Autodesk Inventor part; units mm, degrees
ref_plane "YZ Plane" through (0, 0, 0) normal (1, 0, 0) x (0, 1, 0)
ref_plane "XZ Plane" through (0, 0, 0) normal (0, 1, 0) x (-1, 0, 0)
ref_plane "XY Plane" through (0, 0, 0) normal (0, 0, 1) x (1, 0, 0)
sketch "スケッチ1" plane through (0, 0, 0) normal (0, 1, 0) x (-1, 0, 0)
  circle A0 centre (0, 0) radius 122.5
  line L0 (0, 0) -> (21.2719, 120.6389)
  line L1 (21.2719, 120.6389) -> (-21.2719, -120.6389)
  line L2 (21.2719, 120.6389) -> (-41.166, -233.4643)
  arc A1 (21.2719, 120.6389) -> (0, 122.5) centre (0, 0) ccw
  arc A2 (-21.2719, -120.6389) -> (0, -122.5) centre (0, 0) ccw
  arc A3 (-41.8975, -115.1123) -> (-21.2719, -120.6389) centre (0, 0) ccw
  circle A4 centre (0, 0) radius 125
  circle A5 centre (0, 0) radius 145
  arc A6 (-42.7525, -117.4616) -> (-105.9051, -66.4011) centre (0, 0) ccw
  line L3 (0, 0) -> (-42.7525, -117.4616) construction
  line L4 (21.706, 123.101) -> (21.706, 123.101)
  line L5 (0, -145) -> (0, -265.735)
  line L6 (0, 0) -> (-41.8975, -115.1123)
  line L7 (-49.5929, -136.2554) -> (-41.8975, -115.1123)
  line L8 (-42.7525, -117.4616) -> (-231.4975, -48.764)
  line L9 (42.7525, 117.4616) -> (0, 0)
  line L10 (0, -145) -> (0, 145)
  line L11 (0, 0) -> (0, 250)
  circle A7 centre (0, 250) radius 20
  line L12 (113.4405, 52.5) -> (18.1505, 258.4)
  line L13 (0, 0) -> (185.4327, 0)
  line L14 (0, 0) -> (-259.4726, 94.4403)
  line L15 (42.7525, 117.4616) -> (-253.7236, 225.3701)
  line L16 (0, 125) -> (22.0409, 125)
  line L17 (21.2719, 120.6389) -> (25.179, 142.7971)
  line L18 (42.7525, 117.4616) -> (60.6365, 166.5974)
  line L19 (15, 170) -> (59.0618, 170)
  line L20 (15.9946, 175) -> (56.7478, 175)
  line L21 (0, 125) -> (-15, 125)
  line L22 (-15, 125) -> (-15, 275)
  line L23 (-15, 275) -> (0, 275)
  line L24 (0, 275) -> (0, 125)
  line L25 (0, 125) -> (15, 125)
  line L26 (15, 125) -> (15, 275)
  line L27 (15, 275) -> (0, 275)
  line L28 (0, 275) -> (0, 125)
  line L29 (15, 200) -> (15, 275)
  line L30 (15, 275) -> (-15, 275)
  line L31 (-15, 275) -> (-15, 150)
  line L32 (15, 170) -> (37.5, 170)
  line L33 (37.5, 170) -> (17.5, 170)
  line L34 (0, 0) -> (0, 250)
  line L35 (0, -125) -> (42.7525, 117.4616)
  line L36 (-42.7525, -117.4616) -> (0, 125)
  line L37 (0, -125) -> (-3.519, -144.9573)
  line L38 (42.7525, 117.4616) -> (49.5929, 136.2554)
  line L39 (0, 125) -> (3.519, 144.9573)
  line L40 (-42.7525, -117.4616) -> (-46.2715, -137.4189)
  line L41 (42.7525, 117.4616) -> (46.2715, 137.4189)
  line L42 (-3.519, -144.9573) -> (46.2715, 137.4189)
  line L43 (46.2715, 137.4189) -> (37.2054, 139.0175)
  line L44 (-12.5852, -143.3587) -> (-3.519, -144.9573)
  line L45 (-46.2715, -137.4189) -> (3.519, 144.9573)
  line L46 (3.519, 144.9573) -> (12.5852, 143.3587)
  line L47 (-37.2054, -139.0175) -> (-46.2715, -137.4189)
  line L48 (-27.6373, -142.3418) -> (-22.7132, -143.21)
  line L49 (-27.6373, -142.3418) -> (-22.7132, -143.21)
  line L50 (-22.7132, -143.21) -> (27.641, 142.363)
  line L51 (27.641, 142.363) -> (22.717, 143.2312)
  line L52 (22.717, 143.2312) -> (-27.6373, -142.3418)
  line L53 (12.5852, 143.3587) -> (-37.2054, -139.0175)
  line L54 (-12.5852, -143.3587) -> (37.2054, 139.0175)
  line L55 (-42.1294, -138.1492) -> (7.6611, 144.2269)
  line L56 (-7.6611, -144.2269) -> (42.1294, 138.1492)
  line L57 (12.5852, 143.3587) -> (7.6611, 144.2269)
  line L58 (7.6611, 144.2269) -> (23.8851, 236.2374)
  line L59 (23.8851, 236.2374) -> (28.8091, 235.3692)
  line L60 (28.8091, 235.3692) -> (12.5852, 143.3587)
  line L61 (22.717, 143.2312) -> (25.179, 142.7971)
  line L62 (25.179, 142.7971) -> (42.462, 240.8141)
  line L63 (42.462, 240.8141) -> (40, 241.2482)
  line L64 (40, 241.2482) -> (22.717, 143.2312)
  line L65 (42.1294, 138.1492) -> (37.2054, 139.0175)
  line L66 (37.2054, 139.0175) -> (45.9435, 188.5741)
  line L67 (45.9435, 188.5741) -> (50.8676, 187.7058)
  line L68 (50.8676, 187.7058) -> (42.1294, 138.1492)
  line L69 (25.179, 142.7971) -> (27.641, 142.363)
  line L70 (27.641, 142.363) -> (39.8383, 211.5375)
  line L71 (39.8383, 211.5375) -> (37.3763, 211.9716)
  line L72 (37.3763, 211.9716) -> (25.179, 142.7971)
  line L73 (15.9946, 175) -> (15, 175)
  line L74 (15, 175) -> (0, 175)
  line L75 (0, 175) -> (0, 170)
  line L76 (0, 170) -> (15, 170)
  line L77 (15, 170) -> (15, 175)
  line L78 (20, 175) -> (40, 175)
  line L79 (40, 175) -> (40, 245)
  line L80 (40, 245) -> (20, 245)
  line L81 (20, 245) -> (20, 175)
  line L82 (30, 175) -> (30, 118.7697)
  line L83 (0, 175) -> (45.1779, 175)
  line L84 (45.1779, 175) -> (45.1779, 200)
  line L85 (45.1779, 200) -> (0, 200)
  line L86 (0, 200) -> (0, 175)
  line L87 (0, 200) -> (50, 200)
  line L88 (50, 200) -> (50, 170)
  line L89 (50, 170) -> (0, 170)
  line L90 (0, 170) -> (0, 200)
  line L91 (50, 170) -> (0, 170)
  line L92 (0, 170) -> (0, 165)
  line L93 (0, 200) -> (-15, 200)
  line L94 (-15, 200) -> (-15, 180)
  line L95 (-15, 180) -> (0, 180)
  line L96 (0, 180) -> (0, 200)
  line L97 (0, 180) -> (-15, 180)
  line L98 (-15, 180) -> (-15, 175)
  line L99 (-15, 175) -> (0, 175)
  line L100 (0, 175) -> (0, 180)
  line L101 (0, 145) -> (-15, 145)
  line L102 (-15, 145) -> (-20.5, 145)
  line L103 (-20.5, 145) -> (-20.5, 200)
  line L104 (-20.5, 200) -> (-15, 200)
  line L105 (-15, 200) -> (-15, 145)
  line L106 (-20.5, 150) -> (-25, 150)
  line L107 (-25, 150) -> (-25, 180)
  line L108 (-25, 180) -> (-20.5, 180)
  line L109 (-20.5, 180) -> (-20.5, 150)
  line L110 (50, 175) -> (-15, 175)
  line L111 (-15, 175) -> (-15, 170)
  line L112 (50, 170) -> (50, 175)
  line L113 (-20.5, 165) -> (-25, 165)
  line L114 (-25, 165) -> (-25, 195)
  line L115 (-25, 195) -> (-20.5, 195)
  line L116 (-20.5, 195) -> (-20.5, 165)
  line L117 (15, 250) -> (-15, 250)
  line L118 (-15, 145) -> (15, 145)
  line L119 (26.3471, 235.8033) -> (-39.6674, -138.5834)
  line L120 (48.4056, 188.14) -> (-10.1232, -143.7928)
  line L121 (49.3441, 179.0659) -> (14.8758, 185.1436)
  line L122 (-15, 138.4818) -> (-15, 121.5782)
  line L123 (-7.6611, -144.2269) -> (-42.1294, -138.1492)
  line L124 (-39.6243, -123.9424) -> (-5.1561, -130.02)
  line L125 (-42.2291, -138.7145) -> (-7.7608, -144.7922)
  line L126 (-41.3608, -133.7904) -> (-6.8926, -139.8681)
  line L127 (-6.0243, -134.9441) -> (-40.4926, -128.8664)
  line L128 (18.3488, 204.8397) -> (52.8171, 198.762)
  line L129 (50.2124, 183.9899) -> (45.0029, 154.4457)
  line L130 (10.5346, 160.5234) -> (15.7441, 190.0676)
  line L131 (19.217, 209.7638) -> (53.6853, 203.6861)
  line L132 (15, 250) -> (53.6853, 203.6861)
  line L133 (53.6853, 203.6861) -> (53.6853, 170)
  line L134 (53.6853, 170) -> (-15, 170)
  line L135 (-15, 172.5) -> (53.6853, 172.5)
  line L136 (15, 170) -> (15, 150)
  line L137 (15, 150) -> (-15, 150)
  line L138 (-15, 170) -> (15, 170)
  line L139 (15, 150) -> (-15, 150)
  line L140 (-15, 150) -> (-15, 275)
  line L141 (-15, 275) -> (15, 275)
  line L142 (15, 275) -> (15, 150)
  circle A8 centre (0, 250) radius 6
  circle A9 centre (0, 250) radius 11
  line L143 (47.7456, 170) -> (15, 150)
  point P0 (-25.1752, -142.7759)
  point P1 (42.3116, 114.9608)
  point P2 (0, 133.0222)
  point P3 (-38.8988, -134.2246)
  point P4 (-38.0306, -129.3005)
  point P5 (-23.2585, -131.9052)
  point P6 (-24.1267, -136.8293)
  point P7 (-9.3546, -139.434)
  point P8 (-8.4863, -134.51)
  point P9 (17.3379, 184.7094)
  point P10 (32.11, 182.1047)
  point P11 (46.8821, 179.5)
  point P12 (50.3551, 199.1962)
  point P13 (35.5829, 201.8009)
  point P14 (20.8108, 204.4056)
  point P15 (0, 240)
  point P16 (0, 190)
  point P17 (0, 239)
  point P18 (0, 261)
  point P19 (37.5, 172.5)
  point P20 (22.5, 172.5)
  point P21 (0, 275)
  point P22 (15, 185.1217)
  point P23 (15, 185.8477)
  point P24 (-11, 250)
  point P25 (11, 250)
  dimension "d0" = 245
  dimension "d7" = 290
  dimension "d19" = 40
  dimension "d1" = 0
  dimension "d4" = 42.5438
  dimension "d5" = 21.3532
  dimension "d6" = 250
  dimension "d10" = 0
  dimension "d12" = 0
  dimension "d13" = 10
  dimension "d15" = 0
  dimension "d16" = 9.8877
  dimension "d18" = 10
  dimension "d21" = 145
  dimension "d23" = 125
  dimension "d26" = 7.5384
  dimension "d30" = 180
  dimension "d34" = 180
  dimension "d35" = 45
  dimension "d37" = 5
  dimension "d38" = 15
  dimension "d39" = 150
  dimension "d40" = 15
  dimension "d41" = 150
  dimension "d47" = 250
  dimension "d52" = 5
  dimension "d53" = 0
  dimension "d54" = 10
  dimension "d55" = 10
  dimension "d56" = 5
  dimension "d57" = 5
  dimension "d60" = 5
  dimension "d61" = 20
  dimension "d62" = 70
  dimension "d63" = 5
  dimension "d65" = 25
  dimension "d66" = 50
  dimension "d68" = 20
  dimension "d69" = 5
  dimension "d74" = 20
  dimension "d75" = 5.5
  dimension "d76" = 55
  dimension "d77" = 4.5
  dimension "d78" = 30
  dimension "d79" = 5
  dimension "d82" = 15
  dimension "d83" = 50
  dimension "d87" = 16.9036
  dimension "d88" = 10.0392
  dimension "d89" = 10.5222
  dimension "d92" = 15
  dimension "d93" = 5
  dimension "d94" = 5
  dimension "d96" = 4.5
  dimension "d97" = 5
  dimension "d98" = 30
  dimension "d99" = 10
  dimension "d101" = 20
  dimension "d102" = 10
  dimension "d103" = 20
  dimension "d104" = 12
  dimension "d105" = 22
  dimension "d106" = 7.5
  dimension "d107" = 15
  dimension "d108" = 30
extrude "押し出し1" add sketch "スケッチ1" along normal blind 30 contours L137 L60 L26 | L60 L137 L119 L76 L26 | L76 L119 L26 | L137 L58 L76 L119 | L119 L76 L58 L135 L26 | L137 L11 L76 L58 | L26 L117 A9 L24 A7 | A7 L24 L27 L26 | L137 L22 L134 L11 | L135 L58 L74 L26 | L76 L11 L135 L58 | L24 A9 L117 L22 A7 | A7 L22 L23 L24 | L26 A7 L11 A9 L117 | L74 L58 L121 L26 | L135 L11 L74 L58 | L134 L22 L135 L11 | L26 L85 L11 A7 | A9 L117 A8 L24 | L24 A8 L117 A9 | A9 L11 A8 L117 | L121 L58 L26 | L74 L11 L85 L26 L58 | L135 L22 L99 L11 | A7 L22 L117 A9 L11 | L11 L93 L22 A7 | L117 A8 L11 A9 | L99 L22 L95 L11 | L11 L95 L22 L93
shell "シェル1" thickness 2 removed faces 3 at (-5, 10, 275) at (-5.9805, 20, 249.5172) at (5, 10, 150)
sketch "スケッチ3" plane through (0, 0, 0) normal (0, -1, 0) x (1, 0, 0)
  line L0 (15, 150) -> (-15, 150)
  line L1 (-13, 150) -> (-13, 275)
  point P0 (0, 0)
  point P1 (0, 165)
  point P2 (0, 150)
  point P3 (0, 240)
  point P4 (0, 185)
  point P5 (0, 205)
  point P6 (0, 225)
  dimension "d119" = 15
  dimension "d120" = 0
  dimension "d146" = 20
  dimension "d147" = 20
  dimension "d148" = 13
  dimension "d151" = 20
hole "穴1" at (0, 0, 239) at (0, 0, 261) direction (0, 1, 0) diameter 5 end through all
hole "穴2" at (0, 0, 165) at (0, 0, 240) at (0, 0, 205) at (0, 0, 185) at (0, 0, 225) direction (0, 1, 0) diameter 3.1 end through all
sketch "スケッチ4" plane through (-15, 0, 150) normal (-1, 0, 0) x (0, 0, 1)
  line L0 (0, 0) -> (0, 30)
  line L1 (0, 15) -> (125, 15)
  line L2 (125, 0) -> (125, 30)
  point P0 (-150, 0)
  point P1 (15, 15)
  point P2 (55, 15)
  dimension "d129" = 15
  dimension "d130" = 40
hole "穴3" at (-15, 15, 165) at (-15, 15, 205) direction (1, 0, 0) diameter 3.1 end through all
sketch "スケッチ6" plane through (-15, 0, 150) normal (-1, 0, 0) x (0, 0, 1)
  circle A0 centre (15, 15) radius 1.55
  circle A1 centre (15, 15) radius 5
  circle A2 centre (55, 15) radius 1.55
  circle A3 centre (55, 15) radius 5
  point P0 (-150, 0)
  dimension "d142" = 10
  dimension "d143" = 10
extrude "押し出し3" cut sketch "スケッチ6" against normal blind 5 contours A0 | A1 | A2 | A3
sketch "スケッチ7" plane through (15, 0, 150) normal (0, 0, -1) x (-1, 0, 0)
  line L0 (2, 2) -> (2, 28)
  line L1 (2, 28) -> (28, 28)
  line L2 (28, 28) -> (28, 2)
  line L3 (28, 2) -> (2, 2)
  line L4 (0, 0) -> (30, 0)
  line L5 (30, 0) -> (30, 30)
  line L6 (0, 30) -> (30, 30)
  line L7 (0, 0) -> (0, 30)
  point P0 (15, 0)
extrude "押し出し4" cut sketch "スケッチ7" against normal blind 7.5
equation "\"d18\" = d13"
properties part number "hand2_03" material "アルミニウム 6061-AHC"
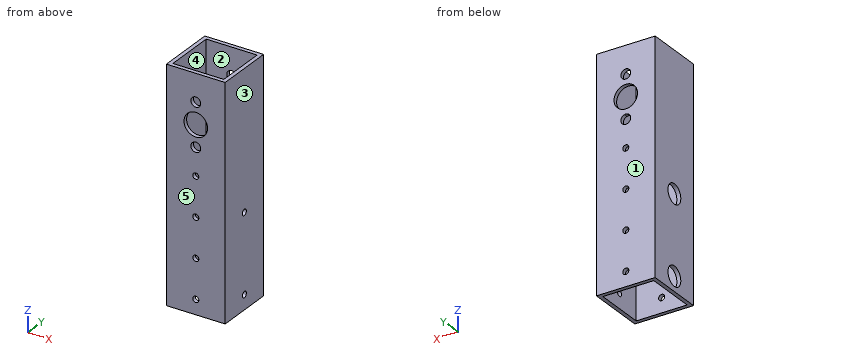
The model under review builds one solid part; all positions refer to its coordinate system, in mm. Face numbers are marked on the shaded views. A direction names the side the tool comes from. Give positions to 0.01 mm unless a question says otherwise; leave off trailing zeros. Write each loop counter-clockwise with the first axis right and the second up, starting at its lowest first coordinate (ties: lowest second). Pieces come first, ordered by that corner, then holes. Notation, with made-up numbers: M 26,88.25 L 37,88.25 A30 ccw 37,124.25 Z; hole C 25,-32 d6. An arc over 180 degrees is marked long. Write each question's results on one line, items separated by ' | '. Start each with the question number.
1. For the marked faces 4 and 5, list the 3-axis set-ups (+Z, -Z, +X, -X, +Y, -Y) from which the entire face can be reached by the end or side of a thin tool; tool diameter is ignored.
2. For probe 1 along X at (y, z) = (10.75, 178.5); probe 2 along Y at (x, z) = (-1.25, 216); probe 3 along Y at (x, z) = (-14.3, 205), list the stretches that pass through material, from the lowest coordinate up. Write a range as [from, to].
3. We need section D-D (x = 7.5). Write out the cut boundary in (y, z), and give its area (3 significant figures).
4. Mouldability with a two-part tool opening along X and no side actions: class the marked faces 1, 2 and 3 as released by +X, released by -X, zero draft, split by the parting line, or undercut.
5. We need section C-C (z = 205). Write out the cut boundary in (x, y).
6. We need section A-A (y = 8). Write out the cut boundary in (x, z), and give its area (3 significant figures).
7. We need section B-B (z = 250). Write out the cut boundary in (x, y), and give its area (3 significant figures).
Results found:
1) face 4: +Z, -Z | face 5: +Z, -Z, +X, -X, -Y
2) probe 1: x = [-15, -13], [13, 15] | probe 2: y = [0, 2], [28, 30] | probe 3: y = [0, 10], [20, 30]
3) outline: M 0,157.5 L 2,157.5 L 2,275 L 0,275 Z; M 28,157.5 L 30,157.5 L 30,275 L 28,275 Z | area: 470 mm^2
4) face 1: zero draft | face 2: undercut | face 3: released by +X
5) outline: M -15,0 L -1.55,0 L -1.55,2 L -13,2 L -13,10 L -15,10 Z; M -15,20 L -13,20 L -13,28 L -1.55,28 L -1.55,30 L -15,30 Z; M 1.55,0 L 15,0 L 15,13.45 L 13,13.45 L 13,2 L 1.55,2 Z; M 1.55,28 L 13,28 L 13,16.55 L 15,16.55 L 15,30 L 1.55,30 Z
6) outline: M -15,157.5 L -13,157.5 L -13,275 L -15,275 Z; M 13,157.5 L 15,157.5 L 15,275 L 13,275 Z | area: 470 mm^2
7) outline: M -15,0 L -6,0 L -6,2 L -13,2 L -13,28 L -6,28 L -6,30 L -15,30 Z; M 6,0 L 15,0 L 15,30 L 6,30 L 6,28 L 13,28 L 13,2 L 6,2 Z | area: 176 mm^2
